Here's how the part is built. I have some questions about the finished solid (model axes, mm). Face numbers are marked on the shaded views. Round coordinates to 2 decimals unless told otherwise and drop trailing zeros. Loops run counter-clockwise (first coordinate to the right, second up) from the corner with the lowest first, then second, coordinate; pieces in that order, holes last. Notation, with made-up numbers: M -1,-24.75 L 52,-24.75 A14 ccw 52,-9.75 Z; hole C 5,58 d10. An arc over 180 degrees is marked long. Use a Markdown table: item, result.
Autodesk Inventor part; units mm, degrees
ref_plane "YZ Plane" through (0, 0, 0) normal (1, 0, 0) x (0, 1, 0)
ref_plane "XZ Plane" through (0, 0, 0) normal (0, 1, 0) x (-1, 0, 0)
ref_plane "XY Plane" through (0, 0, 0) normal (0, 0, 1) x (1, 0, 0)
sketch "Sketch1" plane through (0, 0, 0) normal (0, 0, 1) x (1, 0, 0)
  circle A0 centre (0, 0) radius 33.655
  dimension "d0" = 67.31
extrude "Extrusion1" add sketch "Sketch1" along normal blind 2.54
sketch "Sketch2" plane through (0, 0, 0) normal (0, 0, -1) x (-1, 0, 0)
  circle A0 centre (0, 12.3825) radius 1.8415
  point P0 (0, 0)
  dimension "d3" = 3.683
  dimension "d4" = 12.3825
extrude "Extrusion2" cut sketch "Sketch2" against normal through all
chamfer "Chamfer1" distance 1.27 angle 45 1 edges at (1.8415, 12.3825, 0)
pattern_circular "Circular Pattern1" count 3 over 360 about axis through (0, 0, 0) along (0, 0, 1) of "Extrusion2", "Chamfer1"
sketch "Sketch3" plane through (0, 0, 2.54) normal (0, 0, 1) x (1, 0, 0)
  circle A0 centre (0, 0) radius 7.9375
  circle A1 centre (0, 0) radius 3.4925
  circle A2 centre (0, 0) radius 4.8641
  dimension "d13" = 15.875
  dimension "d14" = 6.985
  dimension "d15" = 9.7282
extrude "Extrusion3" add sketch "Sketch3" along normal blind 6.985 contours A0
extrude "Extrusion4" cut sketch "Sketch3" against normal through all contours A1
fillet "Fillet1" radius 1.27 1 edges at (-7.9375, 0, 2.54)
sketch "Sketch4" plane through (0, 0, 0) normal (0, 0, -1) x (-1, 0, 0)
  line L0 (0, 0) -> (15.3979, 8.89) construction
  line L1 (0, 0) -> (17.78, 0) construction
  circle A0 centre (15.3979, 8.89) radius 3.175
  dimension "d21" = 17.78
  dimension "d22" = 30
  dimension "d23" = 6.35
extrude "Extrusion5" cut sketch "Sketch4" against normal through all
sketch "Sketch5" plane through (0, 0, 9.525) normal (0, 0, 1) x (1, 0, 0)
  circle A0 centre (0, 0) radius 6.4643
  dimension "d26" = 12.9286
extrude "Extrusion6" cut sketch "Sketch5" against normal blind 1.905
properties part number "SmallSpoolEndFore" material "ABS Plastic"
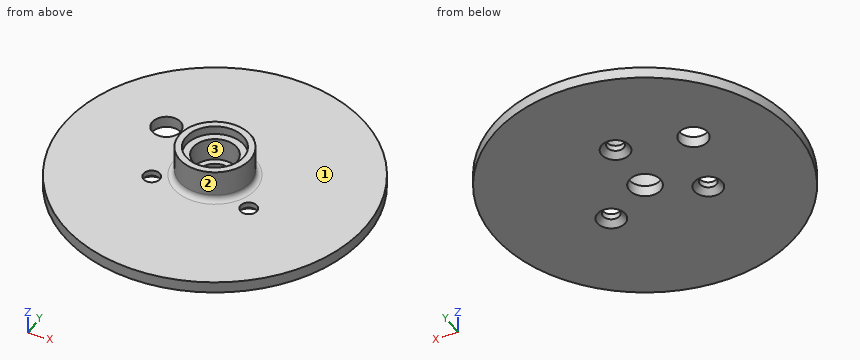
Q1. I need wall thicknesses on line 1 (Y direction, x = 0, z = 1.7) (1 decimal); line 2 (Z direction, x = 25, y = 18.5); line 3 (X direction, y = -3, z = 1.75). Which ranges of each line are inside material? Lowest first, please. Write a range as from..to.
Return value:
| item | result |
|---|---|
| line 1 | y = -33.7..-3.5, 3.5..10.5, 14.2..33.7 |
| line 2 | z = 0..2.54 |
| line 3 | x = -33.52..-1.79, 1.79..33.52 |
Q2. Will these pins go through, and if not, where does the flat tip stop? P1, Ø6.5, axis at x = 2, y = -0.5, coming from the +Z side; P2, Ø3, axis at x = -19, z = 1, coming from the +Y side; P3, Ø4, axis at x = -10.72, y = -6.19, coming from the +Z side.
Return value:
| item | result |
|---|---|
| P1 | stops at z = 7.62 |
| P2 | stops at y = 28.75 |
| P3 | stops at z = 2.54 |
Q3. Imagine slicing it at A-A, the plane x = 0. Please give me the cut outline in (y, z) (1 decimal).
Return value:
| item | result |
|---|---|
| outline | M -33.7,0 L -3.5,0 L -3.5,2.5 L -4.9,2.5 L -4.9,7.6 L -6.5,7.6 L -6.5,9.5 L -7.9,9.5 L -7.9,3.8 A1.3 cw -9.2,2.5 L -33.7,2.5 Z; M 3.5,0 L 9.3,0 L 10.5,1.3 L 10.5,2.5 L 9.2,2.5 A1.3 cw 7.9,3.8 L 7.9,9.5 L 6.5,9.5 L 6.5,7.6 L 4.9,7.6 L 4.9,2.5 L 3.5,2.5 Z; M 14.2,1.3 L 15.5,0 L 33.7,0 L 33.7,2.5 L 14.2,2.5 Z |
Q4. We'd pull the mould along X, two halves only. Please class the marked faces 1, 2 and 3: pulls with the +X half, pulls with the -X half, needs draft (parallel to the pull), parting line crosses it, or undercut.
Return value:
| item | result |
|---|---|
| face 1 | needs draft |
| face 2 | parting line crosses it |
| face 3 | undercut |
Q5. Imagine slicing it at C-C, the plane z = 6.75. Please give me the cut outline in (x, y) (1 decimal).
Return value:
| item | result |
|---|---|
| outline | C 0,0 d15.9; hole C 0,0 d9.7 |
Q6. Imagine slicing it at B-B, the plane y = 0. Please give me the cut outline in (x, z) (1 decimal), then the cut area to 3 significant figures.
Return value:
| item | result |
|---|---|
| outline | M -33.7,0 L -3.5,0 L -3.5,2.5 L -4.9,2.5 L -4.9,7.6 L -6.5,7.6 L -6.5,9.5 L -7.9,9.5 L -7.9,3.8 A1.3 cw -9.2,2.5 L -33.7,2.5 Z; M 3.5,0 L 33.7,0 L 33.7,2.5 L 9.2,2.5 A1.3 cw 7.9,3.8 L 7.9,9.5 L 6.5,9.5 L 6.5,7.6 L 4.9,7.6 L 4.9,2.5 L 3.5,2.5 Z |
| area | 191 mm^2 |
Q7. Imagine slicing it at D-D, the plane x = -22. Please give me the cut outline in (y, z).
Return value:
| item | result |
|---|---|
| outline | M -25.47,0 L 25.47,0 L 25.47,2.54 L -25.47,2.54 Z |
